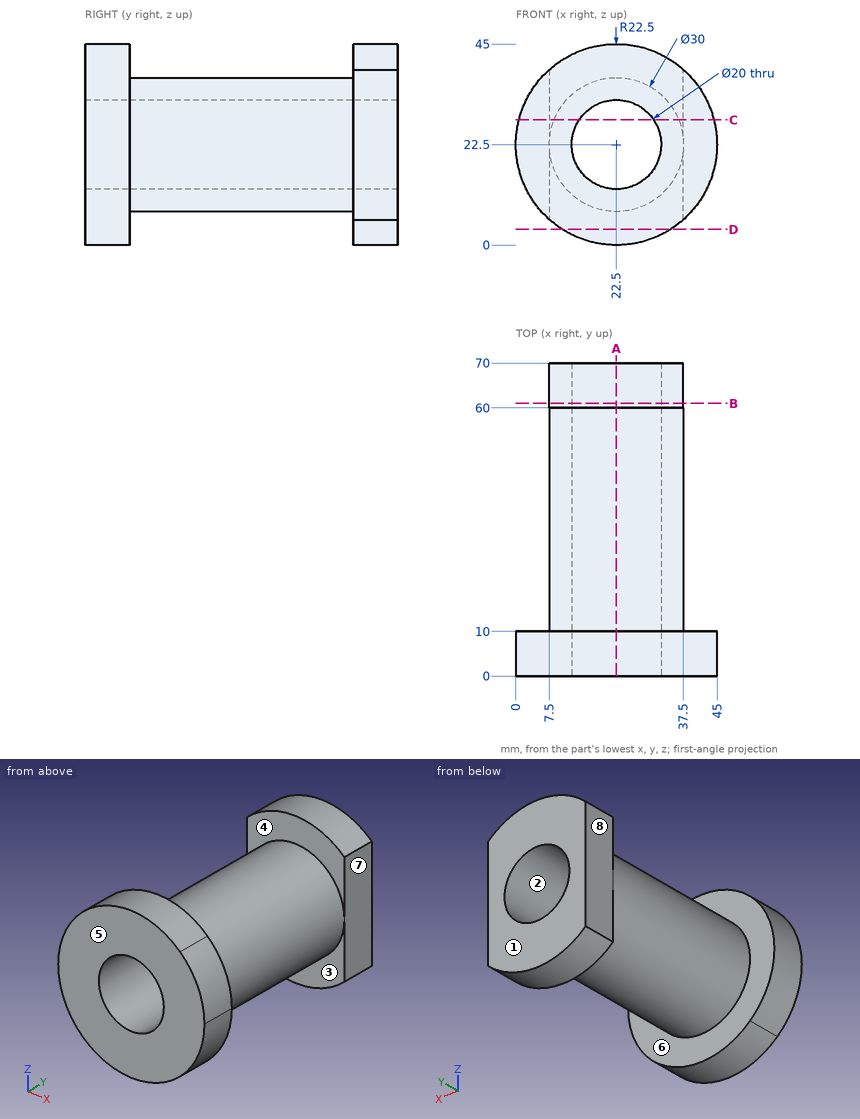
Source: three-view drawing plus pictorial views. Frame: mm from the lowest corner of the part. A direction names the side the tool comes from. Coordinates: 2 decimals unless noted, no trailing zeros. Order: outer loops, then holes, each group sorted by start corner. A loop starts at its lowest first (then second) coordinate and runs counter-clockwise, first axis right, second up. Notation, with made-up numbers: M 72,27.25 L 100,27.25 A8 ccw 100,41.25 Z; hole C 78,-30.75 d7. An arc over 180 degrees is marked long. Write each question's results on one line, items separated by ' | '. Start each with the question number.
1. Section B-B, the plane y = 61. Return the cut outline in (x, z), then the cut area to 3 significant figures.
2. Section C-C, the plane z = 28. Return the cut outline in (x, y).
3. Pin query (flat end, axial travel): pin 1 (11.5 mm diameter, centred on x = 27.5, z = 14.5, fed in from -Y); pin 2 (3 mm diameter, centred on y = 12.5, z = 20.5, fed in from -X); pin 3 (2 mm diameter, centred on y = 8, z = 34, fed in from -X); pin 4 (3 mm diameter, centred on y = 65, z = 29.5, fed in from +X). Return the tip coordinate at first contact, or that it passes through.
4. Section A-A, the plane x = 22.5. Return the cut outline in (y, z).
5. Reachability of the marked faces 4, 5, 6, 7 and 8 from +Z, -Z, +X, -X, +Y, -Y: full face, straight path, thin tool, end or side. Return the list, or none.
6. Material intervals for L1, parallel to Y at x = 17.5, z = 3; L2, parallel to X at y = 33, z = 22; L3, parallel to Y at x = 41, z = 12, sorted ascending.
7. Draft query along Y for the marked faces 1, 2 and 3. Return one class per face: +Y half, -Y half, draft (parallel to the pull), parting line (faces both ways), or undercut.
8. Section D-D, the plane z = 3.5. Return the cut outline in (x, y).
Solution:
1) outline: M 7.5,5.73 A22.5 ccw 37.5,5.73 L 37.5,39.27 A22.5 ccw 7.5,39.27 Z; hole C 22.5,22.5 d20 | area: 928 mm²
2) outline: M 0.68,0 L 14.15,0 L 14.15,70 L 7.5,70 L 7.5,60 L 8.54,60 L 8.54,10 L 0.68,10 Z; M 30.85,0 L 44.32,0 L 44.32,10 L 36.46,10 L 36.46,60 L 37.5,60 L 37.5,70 L 30.85,70 Z
3) pin 1: y = 0 | pin 2: x = 7.51 | pin 3: x = 2.6 | pin 4: x = 37.5
4) outline: M 0,0 L 10,0 L 10,7.5 L 60,7.5 L 60,0 L 70,0 L 70,12.5 L 0,12.5 Z; M 0,32.5 L 70,32.5 L 70,45 L 60,45 L 60,37.5 L 10,37.5 L 10,45 L 0,45 Z
5) face 4: +Z | face 5: +Z, -Z, +X, -X, -Y | face 6: none | face 7: +Z, -Z, +X, +Y | face 8: +Z, -Z, -X, +Y
6) L1: 0 to 10, 60 to 70 | L2: 7.51 to 12.51, 32.49 to 37.49 | L3: 0 to 10
7) face 1: +Y half | face 2: draft | face 3: undercut
8) outline: M 10.45,0 L 34.55,0 L 34.55,10 L 10.45,10 Z; M 10.45,60 L 34.55,60 L 34.55,70 L 10.45,70 Z
